```python
from build123d import *

# Parameters (mm, degrees)
SKETCH1_R           = 30
SKETCH1_R_2         = 12.5
BOSS_EXTRUDE1_DEPTH = 4
SKETCH2_R           = 40
SKETCH2_R_2         = 2.25
SKETCH2_R_3         = 1.5
BOSS_EXTRUDE2_DEPTH = 4
SKETCH3_R           = 3.5
CUT_EXTRUDE1_DEPTH  = 2.5
SKETCH4_R           = 5.15
SKETCH4_R_2         = 2.65
CUT_EXTRUDE2_DEPTH  = 3
SKETCH5_R           = 3.5
BOSS_EXTRUDE3_DEPTH = 0.2


with BuildPart() as part:
    # Sketch1 → Boss-Extrude1 (new body)
    with BuildSketch(Plane.XY):
        Circle(SKETCH1_R)
        Circle(SKETCH1_R_2, mode=Mode.SUBTRACT)
    extrude(amount=BOSS_EXTRUDE1_DEPTH)

    # Sketch2 → Boss-Extrude2 (add)
    with BuildSketch(Plane.XY.offset(4)):
        Circle(SKETCH2_R)
        Circle(SKETCH2_R_2, mode=Mode.SUBTRACT)
        with Locations((-5.655999742, 5.657708628)):
            Circle(SKETCH2_R_3, mode=Mode.SUBTRACT)
        with Locations((-5.655999742, -5.657708628)):
            Circle(SKETCH2_R_3, mode=Mode.SUBTRACT)
        with Locations((5.655999742, -5.657708628)):
            Circle(SKETCH2_R_3, mode=Mode.SUBTRACT)
        with Locations((5.655999742, 5.657708628)):
            Circle(SKETCH2_R_3, mode=Mode.SUBTRACT)
    extrude(amount=BOSS_EXTRUDE2_DEPTH)

    # Sketch3 → Cut-Extrude1 (cut)
    with BuildSketch(Plane.XY.offset(8)):
        with Locations((-5.655999742, 5.657708628)):
            Circle(SKETCH3_R)
        with Locations((5.655999742, 5.657708628)):
            Circle(SKETCH3_R)
        with Locations((5.655999742, -5.657708628)):
            Circle(SKETCH3_R)
        with Locations((-5.655999742, -5.657708628)):
            Circle(SKETCH3_R)
    extrude(amount=-CUT_EXTRUDE1_DEPTH, mode=Mode.SUBTRACT)

    # Sketch4 → Cut-Extrude2 (cut)
    with BuildSketch(Plane(origin=(0, 0, 0), x_dir=(-1, 0, 0), z_dir=(0, 0, -1))):
        with Locations((-20, 0)):
            Circle(SKETCH4_R)
        with Locations((0, -20)):
            Circle(SKETCH4_R)
        with Locations((20, 0)):
            Circle(SKETCH4_R)
        with Locations((0, 20)):
            Circle(SKETCH4_R)
        with Locations((14.142135624, 14.142135624)):
            Circle(SKETCH4_R_2)
        with Locations((14.142135624, -14.142135624)):
            Circle(SKETCH4_R_2)
        with Locations((-14.142135624, -14.142135624)):
            Circle(SKETCH4_R_2)
        with Locations((-14.142135624, 14.142135624)):
            Circle(SKETCH4_R_2)
    extrude(amount=-CUT_EXTRUDE2_DEPTH, mode=Mode.SUBTRACT)

    # Sketch5 → Boss-Extrude3 (add)
    with BuildSketch(Plane.XY.offset(5.5)):
        with Locations((-5.655999742, 5.657708628)):
            Circle(SKETCH5_R)
        with Locations((5.655999742, 5.657708628)):
            Circle(SKETCH5_R)
        with Locations((-5.655999742, -5.657708628)):
            Circle(SKETCH5_R)
        with Locations((5.655999742, -5.657708628)):
            Circle(SKETCH5_R)
    extrude(amount=-BOSS_EXTRUDE3_DEPTH)


solid = part.part
```
The model under review builds one solid part; all positions refer to its coordinate system, in mm. A direction names the side the tool comes from. Round coordinates to 2 decimals unless told otherwise and drop trailing zeros. Write each loop counter-clockwise with the first axis right and the second up, starting at its lowest first coordinate (ties: lowest second). Pieces come first, ordered by that corner, then holes.
(1) We need section D-D on z = 6.75. Give the boundary of the cut face in (x, y), and give its area (3 significant figures).
(2) Machinability: for faces 1 (the cylindrical face through (-0.29, 2.23, 5.97)), 2 (the flat face through (-6, 6, 5.5)), 3 (the cylindrical face through (4.157, 5.724, 4.641)), which of the approach directions +Z, -Z, +X, -X, +Y, -Y give a long, thin tool a straight path to every point of the face, cutting with its end or side? Answer none if there is none.
(3) Wall thickness on L1, parallel to Y at x = 0, z = 1.55; L2, parallel to X at y = -3.5, z = 7.25; L3, parallel to Y at x = -16.5, z = 1.5: over which ranges is each line inside the solid? List them lowest first.
(4) We need section A-A on x = 0. Give the boundary of the cut face in (y, z), and give its area (3 significant figures).
(5) We need section C-C on z = 1.25. Give the number of separate pieces and of enclosed holes in the cut face, and give its area (3 significant figures).
(6) Insertion check: pin 1 (2 mm diameter, centred on y = 10.5, z = 7, fed in from -X); pin 2 (1.6 mm diameter, centred on x = 13, y = 14, fed in from -Z); pin 3 (5 mm diameter, centred on x = -5.66, y = 5.66, fed in from +Z). Each pin has a flat end and moves straight along its axis. Give the tip position at first contact, or say it passes through.
(7) Mouldability with a two-part tool opening along Y and no side actions: class faces 4 (the flat face through (6, 30, 4)), 5 (the cylindrical face through (-6.41, 2.24, 6.77)), 6 (the cylindrical face through (-8.67, -39.05, 5.97)) as +Y half, -Y half, draft (parallel to the pull), parting line (faces both ways), or undercut.
Findings below:
1. outline: circle Ø80 at (0, 0); hole circle Ø7 at (-5.66, -5.66); hole circle Ø7 at (-5.66, 5.66); hole circle Ø4.5 at (0, 0); hole circle Ø7 at (5.66, -5.66); hole circle Ø7 at (5.66, 5.66)
1. area: 4,860 mm2
2. face 1: +Z, -Z
2. face 2: +Z
2. face 3: -Z
3. L1: y = -30 to -25.15, -14.85 to -12.5, 12.5 to 14.85, 25.15 to 30
3. L2: x = -39.85 to -8.41, -2.9 to 2.9, 8.41 to 39.85
3. L3: y = -25.05 to -15.35, -12.93 to -3.78, 3.78 to 12.93, 15.35 to 25.05
4. outline: (-40, 4) - (-30, 4) - (-30, 0) - (-25.15, 0) - (-25.15, 3) - (-14.85, 3) - (-14.85, 0) - (-12.5, 0) - (-12.5, 4) - (-2.25, 4) - (-2.25, 8) - (-40, 8) - close; (2.25, 4) - (12.5, 4) - (12.5, 0) - (14.85, 0) - (14.85, 3) - (25.15, 3) - (25.15, 0) - (30, 0) - (30, 4) - (40, 4) - (40, 8) - (2.25, 8) - close
4. area: 380 mm2
5. separate pieces: 1
5. enclosed holes: 9
5. area: 1,920 mm2
6. pin 1: stops at x = -38.86
6. pin 2: stops at z = 3
6. pin 3: stops at z = 5.5
7. face 4: draft
7. face 5: undercut
7. face 6: parting line
